from build123d import *

# Parameters (mm, degrees)
F1_DEPTH = 10
F3_DEPTH = 10
F4_R     = 4
F5_DEPTH = 10


with BuildPart() as f1:
    # F0 (on Top) → F1 (new body)
    with BuildSketch(Plane.XY):
        with BuildLine():
            ThreePointArc((0, -3), (-0.87868, -0.87868), (-3, 0))
            Line((-3, 0), (-13, 0))
            ThreePointArc((-13, 0), (-15.12132, -0.87868), (-16, -3))
            Line((-16, -3), (-16, -13))
            ThreePointArc((-16, -13), (-15.12132, -15.12132), (-13, -16))
            Line((-13, -16), (-3, -16))
            ThreePointArc((-3, -16), (-0.87868, -15.12132), (0, -13))
            Line((0, -13), (0, -3))
        make_face()
    extrude(amount=F1_DEPTH)

    # F2 (on face) → F3 (join)
    with BuildSketch(Plane.XY.offset(10)):
        with BuildLine():
            Line((-2, 1), (-14, 1))
            ThreePointArc((-14, 1), (-16.12132, 0.12132), (-17, -2))
            Line((-17, -2), (-17, -14))
            ThreePointArc((-17, -14), (-16.12132, -16.12132), (-14, -17))
            Line((-14, -17), (-2, -17))
            ThreePointArc((-2, -17), (0.12132, -16.12132), (1, -14))
            Line((1, -14), (1, -2))
            ThreePointArc((1, -2), (0.12132, 0.12132), (-2, 1))
        make_face()
    extrude(amount=F3_DEPTH)

    # F4 (on face) → F5 (join)
    with BuildSketch(Plane.XY.offset(20)):
        with Locations((-8, -8)):
            Circle(F4_R)
    extrude(amount=F5_DEPTH)


solid = f1.part
Part model, mm, in its own coordinate system. A direction names the side the tool comes from. Round coordinates to 2 decimals unless told otherwise and drop trailing zeros. Loops run counter-clockwise (first coordinate to the right, second up) from the corner with the lowest first, then second, coordinate; pieces in that order, holes last. Notation, with made-up numbers: (-5, 19) - (51, 19) arc R30 ccw to (51, 58) - close; hole circle Ø11 at (12, 51.5). An arc over 180 degrees is marked (long way). Answer as a JSON object with one key per item and string values.
Item 1: Wall check: L1, parallel to Z at x = -11.5, y = -0.25; L2, parallel to X at y = -3.5, z = 6; L3, parallel to Z at x = -1, y = -0.25. Give the ranges that are in metal, low to high.
Output:
{"L1": "0 to 20", "L2": "-16 to 0", "L3": "10 to 20"}
Item 2: Band-saw the part on D-D on z = 5. List the corners of the cut face in (x, y).
Output:
{"outline": "(-16, -13) arc R3 ccw to (-13, -16) - (-3, -16) arc R3 ccw to (0, -13) - (0, -3) arc R3 ccw to (-3, 0) - (-13, 0) arc R3 ccw to (-16, -3) - close"}
Item 3: Band-saw the part on A-A on y = -8. List the corners of the cut face in (x, z).
Output:
{"outline": "(-17, 10) - (-16, 10) - (-16, 0) - (0, 0) - (0, 10) - (1, 10) - (1, 20) - (-4, 20) - (-4, 30) - (-12, 30) - (-12, 20) - (-17, 20) - close"}
Item 4: Tool access for faces 1 (the face through (-15.14, -15.1, 4.93)), 2 (the face through (-11.2, -10.4, 24.9)), 3 (the face through (-0.86, -0.9, 4.93)), 4 (the face through (-8, 0, 5)), 5 (the face through (-16, -8, 5)): list every direction of +Z, -Z, +X, -X, +Y, -Y with a clear straight run to the whole face (end or side of a thin tool).
Output:
{"face 1": "-Z, -X, -Y", "face 2": "+Z", "face 3": "-Z, +X, +Y", "face 4": "-Z, +X, -X, +Y", "face 5": "-Z, -X, +Y, -Y"}
Item 5: Pin check, flat tips, straight feed: pin 1 (3 mm diameter, centred on x = -14, z = 7, fed in from -Y); pin 2 (5 mm diameter, centred on x = -10, z = 4, fed in from +Y); pin 3 (5 mm diameter, centred on y = -9, z = 3.5, fed in from +X). Stop position of each tip, or through.
Output:
{"pin 1": "y = -16", "pin 2": "y = 0", "pin 3": "x = 0"}
Item 6: Band-saw the part on B-B on z = 18. List the corners of the cut face in (x, y), plus the area to 3 significant figures.
Output:
{"outline": "(-17, -14) arc R3 ccw to (-14, -17) - (-2, -17) arc R3 ccw to (1, -14) - (1, -2) arc R3 ccw to (-2, 1) - (-14, 1) arc R3 ccw to (-17, -2) - close", "area": "316 mm2"}
